Model file for the job. Use its own axes, mm. A direction names the side the tool comes from. Round coordinates to 2 decimals unless told otherwise and drop trailing zeros. Loops run counter-clockwise (first coordinate to the right, second up) from the corner with the lowest first, then second, coordinate; pieces in that order, holes last. Notation, with made-up numbers: M 31.25,-25.75 L 73.25,-25.75 A26 ccw 73.25,-3.75 Z; hole C -23,-15 d1. An arc over 180 degrees is marked long. Use a Markdown table: item, result. Add a question column.
Item 1: Two-plate mould, pull along Y, no slides. Class faces 4 (the flat face through (-39.664, 5, 2)), 5 (the flat face through (-77, -35.933, 2)), 6 (the cylindrical face through (-24.234, 44.316, 2.465)): +Y half, -Y half, draft (parallel to the pull), parting line (faces both ways), or undercut.
Item 2: Saw through at B-B on z = 3.4. Write the cut outline in (x, y), then the cut area to 3 significant figures.
Item 3: Wall check: L1, parallel to Y at x = -58, z = 3.2; L2, parallel to X at y = 8, z = 0.35; L3, parallel to Y at x = -66, z = 1.65. Give the ranges that are in metal, low to high. Write a range as from..to.
Item 4: Tool access for faces 1 (the cylindrical face through (-66.594, 29.519, 2.465)), 2 (the cylindrical face through (-69.634, -16.534, 2.465)), 3 (the flat face through (-67.164, 37, 2)): list every direction of +Z, -Z, +X, -X, +Y, -Y with a clear straight run to the whole face (end or side of a thin tool).
Item 5: Saw through at C-C on y = 25. Write the cut outline in (x, z), then the cut area to 3 significant figures.
Item 6: Saw through at A-A on x = -52. Write the cut outline in (y, z).
Item 7: Pin check, flat tips, straight feed: P1, Ø2, axis at y = 3.5, z = 3.5, coming from the -X side; P2, Ø12, axis at x = -64, y = -26.5, coming from the -Z side. Stop position of each tip, or through.
Item 8: Saw through at D-D on x = -97.5. Write the cut outline in (y, z), then the cut area to 3 significant figures.
```python
from build123d import *

# Parameters (mm, degrees)
F1_DEPTH = 5


with BuildPart() as f1:
    # F0 (on Top) → F1 (new body)
    with BuildSketch(Plane.XY):
        with BuildLine():
            ThreePointArc((-67.163906, 30.917319), (-66.578119, 29.503106), (-65.163906, 28.917319))
            Line((-65.163906, 28.917319), (-39.663906, 28.917319))
            Line((-39.663906, 28.917319), (-39.663906, -19.932681))
            Line((-39.663906, -19.932681), (-69.063906, -19.932681))
            Line((-69.063906, -19.932681), (-69.063906, -17.932681))
            ThreePointArc((-69.063906, -17.932681), (-69.649692, -16.518467), (-71.063906, -15.932681))
            Line((-71.063906, -15.932681), (-88.063906, -15.932681))
            Line((-88.063906, -15.932681), (-126.063906, -15.932681))
            ThreePointArc((-126.063906, -15.932681), (-127.478119, -16.518467), (-128.063906, -17.932681))
            Line((-128.063906, -17.932681), (-128.063906, -33.932681))
            ThreePointArc((-128.063906, -33.932681), (-127.478119, -35.346894), (-126.063906, -35.932681))
            Line((-126.063906, -35.932681), (-39.663906, -35.932681))
            Line((-39.663906, -35.932681), (-25.663906, -35.932681))
            ThreePointArc((-25.663906, -35.932681), (-24.249692, -35.346894), (-23.663906, -33.932681))
            Line((-23.663906, -33.932681), (-23.663906, -19.932681))
            Line((-23.663906, -19.932681), (-23.663906, 28.917319))
            Line((-23.663906, 28.917319), (-23.663906, 42.917319))
            ThreePointArc((-23.663906, 42.917319), (-24.249692, 44.331533), (-25.663906, 44.917319))
            Line((-25.663906, 44.917319), (-65.163906, 44.917319))
            ThreePointArc((-65.163906, 44.917319), (-66.578119, 44.331533), (-67.163906, 42.917319))
            Line((-67.163906, 42.917319), (-67.163906, 30.917319))
        make_face()
    extrude(amount=F1_DEPTH)


solid = f1.part
```
Entries:
| question | item | result |
|---|---|---|
| 1 | face 4 | undercut |
| 1 | face 5 | -Y half |
| 1 | face 6 | +Y half |
| 2 | outline | M -128.06,-33.93 A2 ccw -126.06,-35.93 L -25.66,-35.93 A2 ccw -23.66,-33.93 L -23.66,42.92 A2 ccw -25.66,44.92 L -65.16,44.92 A2 ccw -67.16,42.92 L -67.16,30.92 A2 ccw -65.16,28.92 L -39.66,28.92 L -39.66,-19.93 L -69.06,-19.93 L -69.06,-17.93 A2 ccw -71.06,-15.93 L -126.06,-15.93 A2 ccw -128.06,-17.93 Z |
| 2 | area | 3,380 mm2 |
| 3 | L1 | -35.93..-19.93, 28.92..44.92 |
| 3 | L2 | -39.66..-23.66 |
| 3 | L3 | -35.93..-19.93, 29.1..44.73 |
| 4 | face 1 | +Z, -Z, -X |
| 4 | face 2 | +Z, -Z, +Y |
| 4 | face 3 | +Z, -Z, -X, +Y |
| 5 | outline | M -39.66,0 L -23.66,0 L -23.66,5 L -39.66,5 Z |
| 5 | area | 80.0 mm2 |
| 6 | outline | M -35.93,0 L -19.93,0 L -19.93,5 L -35.93,5 Z; M 28.92,0 L 44.92,0 L 44.92,5 L 28.92,5 Z |
| 7 | P1 | x = -39.66 |
| 7 | P2 | z = 0 |
| 8 | outline | M -35.93,0 L -15.93,0 L -15.93,5 L -35.93,5 Z |
| 8 | area | 100 mm2 |
